```python
from build123d import *

# Parameters (mm, degrees)
SKETCH1_R               = 20
BOSS_EXTRUDE1_DEPTH     = 7.25
SKETCH2_R               = 20
SKETCH2_R_2             = 7.5
CUT_EXTRUDE1_DEPTH      = 4.25
CUT_EXTRUDE2_DEPTH      = 32.784430151
CUT_EXTRUDE2_DEPTH_BACK = 32.784430151
SKETCH3_R               = 2.5


with BuildPart() as part:
    # Sketch1 → Boss-Extrude1 (new, symmetric)
    with BuildSketch(Plane(origin=(0, 0, 0), x_dir=(0, 0, -1), z_dir=(1, 0, 0))):
        with Locations(Location((0, 0, 0), (0, 0, 180))):
            Circle(SKETCH1_R)
    extrude(amount=BOSS_EXTRUDE1_DEPTH, both=True)

    # Sketch2 → Cut-Extrude1 (cut, symmetric)
    with BuildSketch(Plane(origin=(0, 0, 0), x_dir=(0, 0, -1), z_dir=(1, 0, 0))):
        with Locations(Location((0, 0, 0), (0, 0, 180))):
            Circle(SKETCH2_R)
        Circle(SKETCH2_R_2, mode=Mode.SUBTRACT)
    extrude(amount=CUT_EXTRUDE1_DEPTH, both=True, mode=Mode.SUBTRACT)

    # Sketch3 → Cut-Extrude2 (cut, two sides: drawn at the far end of the back side and taken through both)
    with BuildSketch(Plane(origin=(7.25, 0, 0), x_dir=(0, 0, -1), z_dir=(1, 0, 0)).offset(-CUT_EXTRUDE2_DEPTH_BACK)):
        Circle(SKETCH3_R)
    extrude(amount=CUT_EXTRUDE2_DEPTH + CUT_EXTRUDE2_DEPTH_BACK, mode=Mode.SUBTRACT)


solid = part.part
```
Work out the finished part from the listing and answer in its coordinate system (mm). A direction names the side the tool comes from. Round coordinates to 2 decimals unless told otherwise and drop trailing zeros. Write each loop counter-clockwise with the first axis right and the second up, starting at its lowest first coordinate (ties: lowest second). Pieces come first, ordered by that corner, then holes.
1) Which of the six approach directions +Z, -Z, +X, -X, +Y, -Y give full straight-line access (tool end or side, diameter ignored) to faces 1 (the face through (-0.059, 0.33, 7.493)), 2 (the face through (-0.1, -2.44, 0.54))?
2) A cutting plane is placed at C-C on x = -5.5. Determine the outline of the cut face in (y, z), and give its area (3 significant figures).
3) A cutting plane is placed at D-D on y = 15. Determine the outline of the cut face in (x, z).
4) Consider probe 1 along X at (y, z) = (10.5, 15.5); probe 2 along Y at (x, z) = (-0.25, 0); probe 3 along Y at (x, z) = (5, -15.5). Determine where each line is inside the solid, lowest interval first.
5) Flat-ended cylindrical pins translate along their axes: P1, Ø3, axis at x = -1, z = -1, coming from the -Y side; P2, Ø1.5, axis at x = 4, y = -14.5, coming from the +Z side; P3, Ø4, axis at x = 5, y = 15, coming from the -Z side. Find the tip coordinate at first contact, or state that the pin passes through.
6) A cutting plane is placed at A-A on z = 0. Determine the outline of the cut face in (x, y).
7) Determine the mould class of faces 3 (the face through (7.25, 0, 4)), 4 (the face through (-5.73, -0.88, -19.98)), 5 (the face through (4.25, 0, 9)) for opening direction X: pulls with the +X half, pulls with the -X half, needs draft (parallel to the pull), parting line crosses it, or undercut.
Entries:
1. face 1: none
1. face 2: +X, -X
2. outline: circle Ø40 at (0, 0); hole circle Ø5 at (0, 0)
2. area: 1,240 mm2
3. outline: (-7.25, -13.23) - (-4.25, -13.23) - (-4.25, 13.23) - (-7.25, 13.23) - close; (4.25, -13.23) - (7.25, -13.23) - (7.25, 13.23) - (4.25, 13.23) - close
4. probe 1: x = -7.25 to -4.25, 4.25 to 7.25
4. probe 2: y = -7.5 to -2.5, 2.5 to 7.5
4. probe 3: y = -12.64 to 12.64
5. P1: stops at y = -7.5
5. P2: stops at z = 14.48
5. P3: stops at z = -15.2
6. outline: (-7.25, -20) - (-4.25, -20) - (-4.25, -7.5) - (4.25, -7.5) - (4.25, -20) - (7.25, -20) - (7.25, -2.5) - (-7.25, -2.5) - close; (-7.25, 2.5) - (7.25, 2.5) - (7.25, 20) - (4.25, 20) - (4.25, 7.5) - (-4.25, 7.5) - (-4.25, 20) - (-7.25, 20) - close
7. face 3: pulls with the +X half
7. face 4: needs draft
7. face 5: undercut
